from build123d import *

# Parameters (mm, degrees)
F3_DEPTH      = 0.3
F4_COUNT      = 4
F5_W          = 0.625
F5_H          = 0.451389
F6_ANGLE_BACK = 90
F6_ANGLE      = 180


with BuildPart() as f1:
    # F0 (on Front) → F1 (revolve)
    with BuildSketch(Plane.XZ):
        with BuildLine():
            Line((0, 20.798611), (0, 0))
            Line((0, 0), (0.555556, 0))
            Line((0.555556, 0), (0.555556, 7.361111))
            Line((0.555556, 7.361111), (0.607639, 7.361111))
            Line((0.607639, 7.361111), (0.607639, 8.055556))
            Line((0.607639, 8.055556), (0.555556, 8.055556))
            Line((0.555556, 8.055556), (0.555556, 20.451389))
            ThreePointArc((0.555556, 20.451389), (0.327569, 20.704666), (0, 20.798611))
        make_face()
    revolve(axis=Axis((0, 0, 10.399306), (0, 0, -1)))

    # F2 (on Front) → F3 (join, symmetric)
    with BuildSketch(Plane.XZ):
        with BuildLine():
            Line((0, 0), (2.048611, 0))
            Line((2.048611, 0), (2.048611, 0.243056))
            ThreePointArc((2.048611, 0.243056), (2.1875, 0.451389), (2.048611, 0.659722))
            Line((2.048611, 0.659722), (2.048611, 2.708333))
            Line((2.048611, 2.708333), (0.4, 4.165245))
            Line((0.4, 4.165245), (0.4, 16.343376))
            Line((0.4, 16.343376), (1.458333, 16.180556))
            Line((1.458333, 16.180556), (0, 19.041132))
            Line((0, 19.041132), (0, 0))
        make_face()
    extrude(amount=F3_DEPTH, both=True)

    # F4: F1 ×4 about axis
    f4_axis = Axis((0, 0, 8.055556), (0, 0, 1))


with BuildPart() as f1_1:
    add(f1.part)
    for i in range(1, F4_COUNT):
        add(f1.part.rotate(f4_axis, i * 360 / F4_COUNT))

    # F5 (on Front) → F6 (revolve)
    with BuildSketch(Plane.XZ, mode=Mode.PRIVATE) as f6_sk:
        with Locations((-0.3125, 13.350694)):
            Rectangle(F5_W, F5_H)
    revolve(f6_sk.sketch.rotate(Axis((0, 0, 8.055556), (0, 0, 1)), -F6_ANGLE_BACK), axis=Axis((0, 0, 8.055556), (0, 0, 1)), revolution_arc=F6_ANGLE)


solid = f1_1.part
The listing builds one solid part. Answer for the finished solid, in the listing's coordinates (mm). A direction names the side the tool comes from. Round coordinates to 2 decimals unless told otherwise and drop trailing zeros. Order: outer loops, then holes, each group sorted by start corner. A loop starts at its lowest first (then second) coordinate and runs counter-clockwise, first axis right, second up. Notation, with made-up numbers: (47, 70) - (71, 70) arc R6 ccw to (71, 78) - close; hole circle Ø3 at (62.5, 21.25). An arc over 180 degrees is marked (long way). Write item = value, one per line. Start each with the question number.
1) Section C-C, the plane x = 1.75 is taken. Write down the section's boundary in (y, z), plus the area to 3 significant figures.
2) For faces 1 (the flat face through (-0.7, -0.3, 16.7)), 2 (the cylindrical face through (0.58, -0.18, 7.71)), determine the directions among +Z, -Z, +X, -X, +Y, -Y from which every point of the face is accessible in a straight line to the end or side of a thin tool.
3) Straight lines are drawn through the part: L1, parallel to Y at x = 0.05, z = 15.25; L2, parallel to Y at x = 1.85, z = 2.75; L3, parallel to Z at x = 0.1, y = -1.3. For each, find the intervals that lie inside material, in ascending order.
4) Section B-B, the plane z = 11.75 is taken. Write down the section's boundary in (x, y).
5) Section A-A, the plane y = -1.25 is taken. Write down the section's boundary in (x, z).
6) Given pin 1 (1 mm diameter, centred on x = 0.5, z = 17, fed in from -Y); pin 2 (1.4 mm diameter, centred on x = -1.5, z = 1.5, fed in from -Y); pin 3 (0.9 mm diameter, centred on y = -1, z = 2.5, fed in from +X), each flat-ended and moving along its own axis, determine where each tip first touches the part or whether it passes through.
7) For a pull along Z with two mould halves and no side action, classify faces 3 (the flat face through (0, 0.97, 17.14)), 4 (the cylindrical face through (-0.555, -0.024, 5.368)), 5 (the flat face through (-0.7, 0.3, 16.7)) as released by +Z, released by -Z, zero draft, split by the parting line, or undercut.
Results list:
q1.outline = (-0.3, 0) - (0.3, 0) - (0.3, 2.97) - (-0.3, 2.97) - close
q1.area = 1.78 mm^2
q2.face_1 = +Z, -X, -Y
q2.face_2 = none
q3.L1 = -0.55 to 0.55
q3.L2 = -0.3 to 0.3
q3.L3 = 0 to 3.37, 16.2 to 16.49
q4.outline = circle Ø1.11 at (0, 0)
q5.outline = (-0.3, 0) - (0.3, 0) - (0.3, 3.41) - (-0.3, 3.41) - close; (-0.3, 16.21) - (0.3, 16.21) - (0.3, 16.59) - (-0.3, 16.59) - close
q6.pin_1 = -1.27
q6.pin_2 = -0.3
q6.pin_3 = 0.3
q7.face_3 = released by +Z
q7.face_4 = undercut
q7.face_5 = zero draft
